For this review, take the finished solid that the model builds, in its own axes (mm). Face numbers are marked on the shaded views. A direction names the side the tool comes from. Round coordinates to 2 decimals unless told otherwise and drop trailing zeros. Order: outer loops, then holes, each group sorted by start corner. A loop starts at its lowest first (then second) coordinate and runs counter-clockwise, first axis right, second up. Notation, with made-up numbers: (-32.75, 8.5) -> (-6.75, 8.5) arc R25 cw to (-6.75, 46.5) -> close; hole circle Ø9 at (-27.5, 56.5). An arc over 180 degrees is marked (long way). Use a Markdown table: item, result. Add a question column.
1) Consider section A-A (x = 0). State the section outline as (y, z) points.
2) Consider section B-B (z = 18). State the section outline as (x, y) points, plus the area to 3 significant figures.
3) Clearance check with flat-ended pins moving along their axes: P1, Ø4, axis at x = -31.18, z = 18, coming from the +Y side; P2, Ø8, axis at x = -31.18, z = -18, coming from the -Y side; P3, Ø8, axis at x = 0, y = -10, coming from the +Z side; P4, Ø5, axis at x = -31, y = 3, coming from the +Z side. State where each tip first meets the part, or that it passes through.
4) Consider section C-C (y = 6.5). State the section outline as (x, z) points.
5) Machinability: for the marked faces 1 and 2, which of the approach directions +Z, -Z, +X, -X, +Y, -Y give a long, thin tool a straight path to every point of the face, cutting with its end or side? Answer none if there is none.
6) Wall thickness on line 1 along Y through (x, z) = (0, 4); line 2 along X through (y, z) = (8, -18); line 3 along Y through (x, z) = (-18.5, 35.5): over which ranges is each line inside the solid? List them lowest first. Write a range as [from, to].
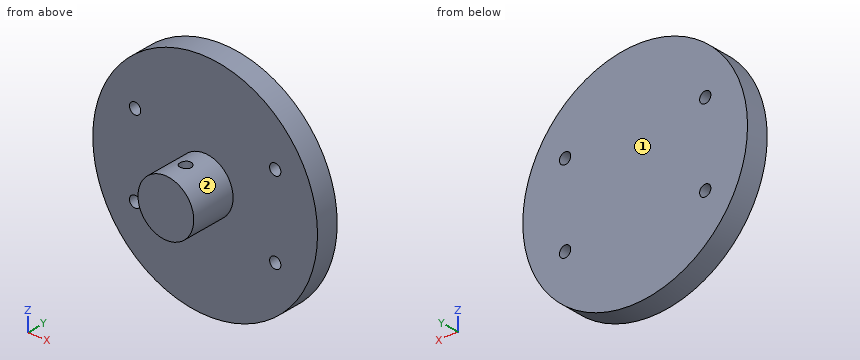
```python
from build123d import *

# Parameters (mm, degrees)
SKETCH2_R               = 50
SKETCH2_R_2             = 2.5
BOSS_EXTRUDE1_DEPTH     = 10
SKETCH3_R               = 12.4125
BOSS_EXTRUDE2_DEPTH     = 20
SKETCH4_R               = 2.5
CUT_EXTRUDE1_DEPTH      = 51
CUT_EXTRUDE1_DEPTH_BACK = 51


with BuildPart() as part:
    # Sketch2 → Boss-Extrude1 (new body)
    with BuildSketch(Plane(origin=(0, 0, 0), x_dir=(1, 0, 0), z_dir=(0, 1, 0))):
        Circle(SKETCH2_R)
        with Locations((-31.176914536, 18)):
            Circle(SKETCH2_R_2, mode=Mode.SUBTRACT)
        with Locations((-31.176914536, -18)):
            Circle(SKETCH2_R_2, mode=Mode.SUBTRACT)
        with Locations((31.176914536, 18)):
            Circle(SKETCH2_R_2, mode=Mode.SUBTRACT)
        with Locations((31.176914536, -18)):
            Circle(SKETCH2_R_2, mode=Mode.SUBTRACT)
    extrude(amount=BOSS_EXTRUDE1_DEPTH)

    # Sketch3 → Boss-Extrude2 (add)
    with BuildSketch(Plane.XZ):
        Circle(SKETCH3_R)
    extrude(amount=BOSS_EXTRUDE2_DEPTH)

    # Sketch4 → Cut-Extrude1 (cut, two sides)
    with BuildSketch(Plane.XY) as cut_extrude1_sk:
        with Locations((0, -10)):
            Circle(SKETCH4_R)
    extrude(amount=CUT_EXTRUDE1_DEPTH, mode=Mode.SUBTRACT)
    extrude(cut_extrude1_sk.sketch, amount=-CUT_EXTRUDE1_DEPTH_BACK, mode=Mode.SUBTRACT)


solid = part.part
```
Results list:
| question | item | result |
|---|---|---|
| 1 | outline | (-20, -12.41) -> (-12.5, -12.41) -> (-12.5, 12.41) -> (-20, 12.41) -> close; (-7.5, -12.41) -> (0, -12.41) -> (0, -50) -> (10, -50) -> (10, 50) -> (0, 50) -> (0, 12.41) -> (-7.5, 12.41) -> close |
| 2 | outline | (-46.65, 0) -> (-33.68, 0) -> (-33.68, 10) -> (-46.65, 10) -> close; (-28.68, 0) -> (28.68, 0) -> (28.68, 10) -> (-28.68, 10) -> close; (33.68, 0) -> (46.65, 0) -> (46.65, 10) -> (33.68, 10) -> close |
| 2 | area | 833 mm2 |
| 3 | P1 | through |
| 3 | P2 | y = 0 |
| 3 | P3 | z = 12.41 |
| 3 | P4 | z = 41.08 |
| 4 | outline | circle Ø100 at (0, 0); hole circle Ø5 at (-31.18, -18); hole circle Ø5 at (-31.18, 18); hole circle Ø5 at (31.18, -18); hole circle Ø5 at (31.18, 18) |
| 5 | face 1 | +Z, -Z, +X, -X, +Y |
| 5 | face 2 | -Y |
| 6 | line 1 | [-20, -12.5], [-7.5, 10] |
| 6 | line 2 | [-46.65, -33.68], [-28.68, 28.68], [33.68, 46.65] |
| 6 | line 3 | [0, 10] |
